Design review of the part built by this model. Coordinates are the model's own, in mm. A direction names the side the tool comes from. Give positions to 0.01 mm unless a question says otherwise; leave off trailing zeros. Order: outer loops, then holes, each group sorted by start corner. A loop starts at its lowest first (then second) coordinate and runs counter-clockwise, first axis right, second up. Notation, with made-up numbers: (41.5, 42) -> (97.5, 42) arc R6 ccw to (97.5, 50) -> close; hole circle Ø11 at (-37.5, 67.25). An arc over 180 degrees is marked (long way). Return JSON: item names as keys, results as strings.
```python
from build123d import *

# Parameters (mm, degrees)
CROQUIS1_R              = 5.125
SALIENTE_EXTRUIR1_DEPTH = 2.6
CROQUIS1_3_R            = 9
CROQUIS1_3_R_2          = 5.125
SALIENTE_EXTRUIR2_DEPTH = 3.1


with BuildPart() as part:
    # Croquis1 → Saliente-Extruir1 (new, symmetric)
    with BuildSketch(Plane.XY):
        with BuildLine():
            ThreePointArc((6.54, -6.182911935), (0, -9), (-6.54, -6.182911935))
            Line((-6.54, -6.182911935), (-6.54, -170.567088065))
            ThreePointArc((-6.54, -170.567088065), (0, -185.75), (6.54, -170.567088065))
            Line((6.54, -170.567088065), (6.54, -6.182911935))
        make_face()
        with Locations((0, -176.75)):
            Circle(CROQUIS1_R, mode=Mode.SUBTRACT)
    extrude(amount=SALIENTE_EXTRUIR1_DEPTH, both=True)

    # Croquis1<3> → Saliente-Extruir2 (add, symmetric)
    with BuildSketch(Plane.XY):
        Circle(CROQUIS1_3_R)
        with Locations(Location((0, 0, 0), (0, 0, 180))):
            Circle(CROQUIS1_3_R_2, mode=Mode.SUBTRACT)
    extrude(amount=SALIENTE_EXTRUIR2_DEPTH, both=True)


solid = part.part
```
Item 1: Add section B-B (x = 0). Give the boundary of the cut face in (y, z) (3 decimals), plus the area to 3 significant figures.
Result set:
{"outline": "(-185.75, -2.6) -> (-181.875, -2.6) -> (-181.875, 2.6) -> (-185.75, 2.6) -> close; (-171.625, -2.6) -> (-9, -2.6) -> (-9, -3.1) -> (-5.125, -3.1) -> (-5.125, 3.1) -> (-9, 3.1) -> (-9, 2.6) -> (-171.625, 2.6) -> close; (5.125, -3.1) -> (9, -3.1) -> (9, 3.1) -> (5.125, 3.1) -> close", "area": "914 mm^2"}
Item 2: Add section C-C (z = -0.75). Give the boundary of the cut face in (x, y) (3 decimals).
Result set:
{"outline": "(-6.54, -170.567) arc R9 ccw (long way) to (6.54, -170.567) -> (6.54, -6.183) arc R9 ccw (long way) to (-6.54, -6.183) -> close; hole circle Ø10.25 at (0, -176.75); hole circle Ø10.25 at (0, 0)"}
Item 3: Add section A-A (y = -176.75). Give the boundary of the cut face in (x, z) (3 decimals).
Result set:
{"outline": "(-9, -2.6) -> (-5.125, -2.6) -> (-5.125, 2.6) -> (-9, 2.6) -> close; (5.125, -2.6) -> (9, -2.6) -> (9, 2.6) -> (5.125, 2.6) -> close"}
Item 4: For pin 1 (3 mm diameter, centred on x = 4.5, z = 1, fed in from +Y); pin 2 (2.5 mm diameter, centred on y = -101, z = 1, fed in from -X); pin 3 (5 mm diameter, centred on x = -1, y = -39.5, fed in from -Z), all flat-tipped, find the tip position at first contact; note any pin that passes through.
Result set:
{"pin 1": "stops at y = 8.49", "pin 2": "stops at x = -6.54", "pin 3": "stops at z = -2.6"}
Item 5: Wall thickness on L1, parallel to Y at x = 0, z = 0.25 (3 decimals); L2, parallel to Y at x = 1.25, z = 2.25; L3, parallel to Z at x = -0.25, y = -118: over which ranges is each line inside the solid? List them lowest first. Write a range as [from, to].
Result set:
{"L1": "y = [-185.75, -181.875], [-171.625, -5.125], [5.125, 9]", "L2": "y = [-185.66, -181.72], [-171.78, -4.97], [4.97, 8.91]", "L3": "z = [-2.6, 2.6]"}
Item 6: Add section D-D (y = -87.5). Give the boundary of the cut face in (x, z).
Result set:
{"outline": "(-6.54, -2.6) -> (6.54, -2.6) -> (6.54, 2.6) -> (-6.54, 2.6) -> close"}
Item 7: Mouldability with a two-part tool opening along X and no side actions: class faces 1 (the face through (-4.734, 1.963, -0.043)), 2 (the face through (4, -4, 3.1)), 3 (the face through (-1.172, 8.923, 0.043)) as released by +X, released by -X, zero draft, split by the parting line, or undercut.
Result set:
{"face 1": "undercut", "face 2": "zero draft", "face 3": "split by the parting line"}
Item 8: Machinability: for faces 4 (the face through (-6.54, -87, 0)), 5 (the face through (6.54, -90, 0)), 6 (the face through (4, -4, -3.1)), which of the approach directions +Z, -Z, +X, -X, +Y, -Y give a long, thin tool a straight path to every point of the face, cutting with its end or side? Answer none if there is none.
Result set:
{"face 4": "+Z, -Z, -X", "face 5": "+Z, -Z, +X", "face 6": "-Z, +X, -X, +Y, -Y"}
